from build123d import *

# Parameters (mm, degrees)
SKETCH1_W            = 70
SKETCH1_H            = 212
SKETCH1_W_2          = 58
SKETCH1_H_2          = 200
BOSS_EXTRUDE1_DEPTH  = 30
SKETCH10_W           = 2
SKETCH10_H           = 6
BOSS_EXTRUDE3_DEPTH  = 16
FILLET2_R            = 3
SKETCH2_R            = 1.5
CUT_EXTRUDE1_DEPTH   = 131.52202895
CUT_EXTRUDE2_REACH   = 218.954
SKETCH3_W            = 12
SKETCH3_H            = 10
SKETCH4_W            = 3
SKETCH4_H            = 1
BOSS_EXTRUDE2_DEPTH  = 16.35
FILLET1_R            = 1.5
SKETCH6_R            = 0.5
CUT_EXTRUDE4_DEPTH   = 120.075910751
FILLET1_OF_MIRROR2_R = 1.5


with BuildPart() as part:
    # Sketch1 → Boss-Extrude1 (new body)
    with BuildSketch(Plane(origin=(0, 0, 0), x_dir=(1, 0, 0), z_dir=(0, 1, 0))):
        Rectangle(SKETCH1_W, SKETCH1_H)
        Rectangle(SKETCH1_W_2, SKETCH1_H_2, mode=Mode.SUBTRACT)
    extrude(amount=BOSS_EXTRUDE1_DEPTH)

    # Sketch7 → Loft3 section 0
    with BuildSketch(Plane.XY.offset(-100)):
        with BuildLine():
            Line((-10, 30), (10, 30))
            Line((10, 30), (10, 27))
            Line((10, 27), (-10, 27))
            Line((-10, 27), (-10, 30))
        make_face()
    # Sketch8 → Loft3 section 1
    with BuildSketch(Plane.XY.offset(-62)):
        with BuildLine():
            Line((-2.5, 30), (2.5, 30))
            Line((2.5, 30), (2.5, 27))
            Line((2.5, 27), (-2.5, 27))
            Line((-2.5, 27), (-2.5, 30))
        make_face()
    loft()

    # Sketch10 → Boss-Extrude3 (add)
    with BuildSketch(Plane.XZ.offset(-27)):
        with Locations((0, -65)):
            Rectangle(SKETCH10_W, SKETCH10_H)
    extrude(amount=BOSS_EXTRUDE3_DEPTH)

    # Fillet2
    fillet2_edges = [part.edges().sort_by_distance(p)[0] for p in [
        (0, 11, -68),
        (0, 11, -62),
    ]]
    fillet(fillet2_edges, radius=FILLET2_R - 0.0001)  # a hair under: the kernel refuses the full size

    # Sketch2 → Cut-Extrude1 (cut, through all)
    with BuildSketch(Plane(origin=(35, 0, 0), x_dir=(0, 0, -1), z_dir=(1, 0, 0))):
        with Locations(Location((65, 15, 0), (0, 0, 270))):
            Circle(SKETCH2_R)
        with Locations((87, 15)):
            Circle(SKETCH2_R)
    extrude(amount=-CUT_EXTRUDE1_DEPTH, mode=Mode.SUBTRACT)

    # Sketch3 → Cut-Extrude2 (cut, up to next)
    with BuildSketch(Plane(origin=(0, 0, -106), x_dir=(-1, 0, 0), z_dir=(0, 0, -1)), mode=Mode.PRIVATE) as cut_extrude2_sk1:
        with Locations((0, 15)):
            Rectangle(SKETCH3_W, SKETCH3_H)
    cut_extrude2_tool1 = extrude(cut_extrude2_sk1.sketch, amount=-CUT_EXTRUDE2_REACH, mode=Mode.PRIVATE) & part.part
    add(cut_extrude2_tool1.solids().sort_by_distance((0, 15, -106))[0], mode=Mode.SUBTRACT)

    # Sketch4 → Boss-Extrude2 (add)
    with BuildSketch(Plane(origin=(35, 0, 0), x_dir=(0, 0, -1), z_dir=(1, 0, 0))):
        with Locations((72.75, 13)):
            Rectangle(SKETCH4_W, SKETCH4_H)
        with Locations((72.75, 17)):
            Rectangle(SKETCH4_W, SKETCH4_H)
    boss_extrude2 = extrude(amount=BOSS_EXTRUDE2_DEPTH)

    # Fillet1
    fillet1_edges = [part.edges().sort_by_distance(p)[0] for p in [
        (51.35, 13, -74.25),
        (51.35, 13, -71.25),
        (51.35, 17, -71.25),
        (51.35, 17, -74.25),
    ]]
    fillet(fillet1_edges, radius=FILLET1_R - 0.0001)  # a hair under: the kernel refuses the full size

    # Sketch6 → Cut-Extrude4 (cut, through all)
    with BuildSketch(Plane(origin=(0, 17.5, 0), x_dir=(1, 0, 0), z_dir=(0, 1, 0))):
        with Locations(Location((49.85, 72.75, 0), (0, 0, 270))):
            Circle(SKETCH6_R)
    cut_extrude4 = extrude(amount=-CUT_EXTRUDE4_DEPTH, mode=Mode.SUBTRACT)

    # Mirror2: Boss-Extrude2, Cut-Extrude4 across plane
    add(boss_extrude2.mirror(Plane(origin=(0, 0, 0), x_dir=(0, 0, 1), z_dir=(1, 0, 0))))
    add(cut_extrude4.mirror(Plane(origin=(0, 0, 0), x_dir=(0, 0, 1), z_dir=(1, 0, 0))), mode=Mode.SUBTRACT)

    # Fillet1 of Mirror2
    fillet1_of_mirror2_edges = [part.edges().sort_by_distance(p)[0] for p in [
        (-51.35, 13, -74.25),
        (-51.35, 13, -71.25),
        (-51.35, 17, -71.25),
        (-51.35, 17, -74.25),
    ]]
    fillet(fillet1_of_mirror2_edges, radius=FILLET1_OF_MIRROR2_R - 0.0001)  # a hair under: the kernel refuses the full size


solid = part.part
The model under review builds one solid part; all positions refer to its coordinate system, in mm. A direction names the side the tool comes from. Give positions to 0.01 mm unless a question says otherwise; leave off trailing zeros. Write each loop counter-clockwise with the first axis right and the second up, starting at its lowest first coordinate (ties: lowest second). Pieces come first, ordered by that corner, then holes.
1. Add section B-B, the plane x = -41. Write out the cut boundary in (y, z).
2. Tool access review of faces 5 (the flat face through (0, 20, -103)), 6 (the flat face through (-6.198, 28.479, -80.734)), 7 (the flat face through (-1, 19, -65)): name each direction out of +Z, -Z, +X, -X, +Y, -Y from which nothing blocks a thin tool from reaching the whole face with its end or side.
3. Wall thickness on L1, parallel to Z at x = 0, y = 15; L2, parallel to X at y = 11.5, z = 19.5; L3, parallel to Y at x = -32, z = -87: over which ranges is each line inside the solid? List them lowest first.
4. Add section A-A, the plane z = 52. Write out the cut boundary in (x, y).
5. Draft analysis for pull direction Z (two halves, no side actions). For faces 1 (the flat face through (29, 15, 1)), 2 (the flat face through (6, 15, -103)), 3 (the flat face through (0, 15, 106)), 4 (the flat face through (1, 19, -65)), state which applies: +Z half, -Z half, draft (parallel to the pull), parting line (faces both ways), or undercut.
6. For P1, Ø12, axis at y = 14.5, z = -46, coming from the +X side; P2, Ø3.5, axis at x = -39, z = -72.5, coming from the +Y side; P3, Ø0.5, axis at x = -41.5, y = 17, coming from the -Z side, all flat-tipped, find the tip position at first contact; note any pin that passes through.
Worked answers:
1. outline: (12.5, -74.25) - (13.5, -74.25) - (13.5, -71.25) - (12.5, -71.25) - close; (16.5, -74.25) - (17.5, -74.25) - (17.5, -71.25) - (16.5, -71.25) - close
2. face 5: -Z
2. face 6: +Y, -Y
2. face 7: -Y
3. L1: z = -68 to -66.5, -63.5 to -62, 100 to 106
3. L2: x = -35 to -29, 29 to 35
3. L3: y = 0 to 13.5, 16.5 to 30
4. outline: (-35, 0) - (-29, 0) - (-29, 30) - (-35, 30) - close; (29, 0) - (35, 0) - (35, 30) - (29, 30) - close
5. face 1: undercut
5. face 2: draft
5. face 3: +Z half
5. face 4: undercut
6. P1: stops at x = 35
6. P2: stops at y = 17.5
6. P3: stops at z = -74.25
